Input: part model. Units: mm. Frame: model coordinates. A direction names the side the tool comes from. Give positions to 0.01 mm unless a question says otherwise; leave off trailing zeros. Loops run counter-clockwise (first coordinate to the right, second up) from the corner with the lowest first, then second, coordinate; pieces in that order, holes last. Notation, with made-up numbers: (-16.5, 7) - (33.5, 7) arc R26 cw to (33.5, 42) - close; hole circle Ø3 at (19, 40.5). An arc over 180 degrees is marked (long way). Answer as a JSON object with one key per item and string values. Group by question number.
(1) Section query B-B (y = 15). Return loops of the section in (x, z), plus the area to 3 significant figures.
(2) Material intervals for L1, parallel to Y at x = 118, z = 7.5; L2, parallel to X at y = 48, z = 11.75; L3, parallel to Y at x = 131, z = 2.75, sorted ascending.
(3) Pin query (flat end, axial travel): P1, Ø6, axis at y = 40.5, z = 6.5, coming from the +X side; P2, Ø10, axis at x = 57.5, z = 18, coming from the +Y side; P3, Ø5, axis at y = 68, z = 9, coming from the +X side. Return the tip coordinate at first contact, or that it passes through.
(4) Access query for faces 4 (the flat face through (111, 57, 12)), 5 (the flat face through (65, 31, 0)), 6 (the flat face through (59, 0, 12)). Directions: +Z, -Z, +X, -X, +Y, -Y. A direction counts if a zero-diameter tool reaches every point of the face in a straight line with its end or side. Return the directions, or none.
(5) Section query C-C (z = 11.5). Return loops of the section in (x, y).
(6) Mould query, pull axis Y, two halves, no side actions, for faces 1 (the flat face through (67, 52, 12)), 2 (the flat face through (34, 33, 12)), 3 (the cylindrical face through (76.014, 84.297, 12.325)). Classes: +Y half, -Y half, draft (parallel to the pull), parting line (faces both ways), or undercut.
(7) Section query A-A (x = 29). Return loops of the section in (y, z), plus the area to 3 significant figures.
```python
from build123d import *

# Parameters (mm, degrees)
EXTRUDE_THIN11_DEPTH = 25


with BuildPart() as part:
    # Sketch2 → Extrude-Thin11 (new body)
    with BuildSketch(Plane.XY):
        with BuildLine():
            Line((67, 70), (67, 33))
            Line((67, 33), (0, 33))
            ThreePointArc((0, 33), (-18, 15), (0, -3))
            Line((0, -3), (120, -3))
            ThreePointArc((120, -3), (138, 15), (120, 33))
            Line((120, 33), (103, 33))
            Line((103, 33), (103, 57))
            Line((103, 57), (120, 57))
            ThreePointArc((120, 57), (138, 75), (120, 93))
            Line((120, 93), (90, 93))
            ThreePointArc((90, 93), (73.736544033, 86.263455967), (67, 70))
        make_face()
        with BuildLine():
            Line((70, 70), (70, 30))
            Line((70, 30), (0, 30))
            ThreePointArc((0, 30), (-15, 15), (0, 0))
            Line((0, 0), (120, 0))
            ThreePointArc((120, 0), (135, 15), (120, 30))
            Line((120, 30), (100, 30))
            Line((100, 30), (100, 60))
            Line((100, 60), (120, 60))
            ThreePointArc((120, 60), (135, 75), (120, 90))
            Line((120, 90), (90, 90))
            ThreePointArc((90, 90), (75.857864376, 84.142135624), (70, 70))
        make_face(mode=Mode.SUBTRACT)
    extrude(amount=EXTRUDE_THIN11_DEPTH)


solid = part.part
```
Recorded:
{
 "1": {"outline": "(-18, 0) - (-15, 0) - (-15, 25) - (-18, 25) - close; (135, 0) - (138, 0) - (138, 25) - (135, 25) - close", "area": "150 mm^2"},
 "2": {"L1": "y = -3 to 0, 30 to 33, 57 to 60, 90 to 93", "L2": "x = 67 to 70, 100 to 103", "L3": "y = 0.75 to 4.8, 25.2 to 29.25, 60.75 to 64.8, 85.2 to 89.25"},
 "3": {"P1": "stops at x = 103", "P2": "stops at y = 33", "P3": "stops at x = 137.43"},
 "4": {"face 4": "+Z, -Z, +X", "face 5": "-Z, +X, -X, +Y, -Y", "face 6": "+Z, -Z"},
 "5": {"outline": "(0, -3) - (120, -3) arc R18 ccw to (120, 33) - (103, 33) - (103, 57) - (120, 57) arc R18 ccw to (120, 93) - (90, 93) arc R23 ccw to (67, 70) - (67, 33) - (0, 33) arc R18 ccw to start; hole (0, 0) - (120, 0) arc R15 ccw to (120, 30) - (100, 30) - (100, 60) - (120, 60) arc R15 ccw to (120, 90) - (90, 90) arc R20 ccw to (70, 70) - (70, 30) - (0, 30) arc R15 ccw to start"},
 "6": {"face 1": "draft", "face 2": "+Y half", "face 3": "undercut"},
 "7": {"outline": "(-3, 0) - (0, 0) - (0, 25) - (-3, 25) - close; (30, 0) - (33, 0) - (33, 25) - (30, 25) - close", "area": "150 mm^2"}
}
